CAD build for the part. Positions are in the model's coordinates, mm. Face numbers are marked on the shaded views. Coordinates: 2 decimals unless noted, no trailing zeros. Order: outer loops, then holes, each group sorted by start corner. A loop starts at its lowest first (then second) coordinate and runs counter-clockwise, first axis right, second up. Notation, with made-up numbers: (-15, -2) -> (7, -2) arc R16 cw to (7, 20) -> close; hole circle Ø8 at (0.5, 3). An arc over 180 degrees is marked (long way). Use one line per item in the form item = value. Start each with the question number.
from build123d import *

# Parameters (mm, degrees)
SKETCH_1_W          = 2
SKETCH_1_H          = 2
SKETCH_2_R          = 1
EXTRUDE_1_DEPTH     = 5
CUT_EXTRUDE_1_DEPTH = 1.5
FILLET_1_R          = 0.3


with BuildPart() as part:
    # 草图1 → 旋转1 (revolve)
    with BuildSketch(Plane.XY):
        with Locations((1, -1)):
            Rectangle(SKETCH_1_W, SKETCH_1_H)
    revolve(axis=Axis((0, 0, 0), (0, -1, 0)))

    # 草图2 → 凸台-拉伸1 (add)
    with BuildSketch(Plane.XZ.offset(2)):
        Circle(SKETCH_2_R)
    extrude(amount=EXTRUDE_1_DEPTH)

    # 草图3 → 切除-拉伸1 (cut)
    with BuildSketch(Plane(origin=(0, 0, 0), x_dir=(-1, 0, 0), z_dir=(0, 1, 0))):
        Polygon((0, -0.866025404), (0.75, -0.433012702), (0.75, 0.433012702), (0, 0.866025404), (-0.75, 0.433012702), (-0.75, -0.433012702), align=None)
    extrude(amount=-CUT_EXTRUDE_1_DEPTH, mode=Mode.SUBTRACT)

    # 圆角1
    fillet_1_edges = [part.edges().sort_by_distance(p)[0] for p in [
        (-1, -7, 0),
        (-2, -2, 0),
        (-2, 0, 0),
    ]]
    fillet(fillet_1_edges, radius=FILLET_1_R)


solid = part.part
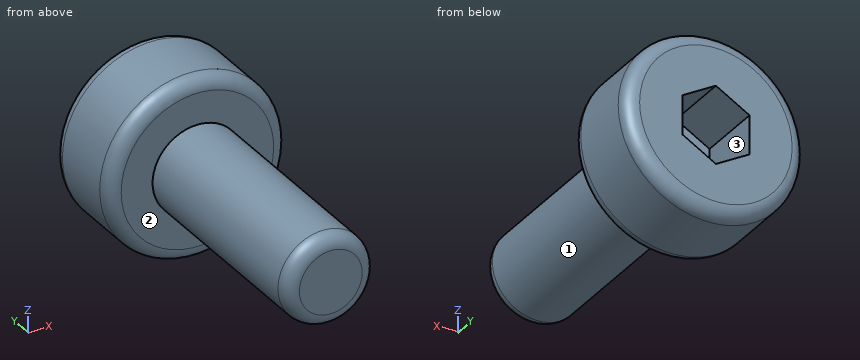
1) Probe L1, parallel to Y at x = -1.45, z = 0.4; L2, parallel to Y at x = -0.45, z = -0.35; L3, parallel to Z at x = -1.05, y = -1. List the from-to ranges inside material, lowest first.
2) Cut at B-B on y = -5. Give the cut face in (x, z).
3) Drop a flat-ended pin along its axis: P1, Ø1, axis at x = 1, y = -6, coming from the +Z side. Give the stop position or say it passes through.
4) Cut at A-A on z = 0. Give the cut face in (x, y).
5) Two-plate mould, pull along X, no slides. Class the marked faces 1, 2 and 3: released by +X, released by -X, zero draft, split by the parting line, or undercut.
Values follow:
q1.L1 = -2 to 0
q1.L2 = -7 to -1.5
q1.L3 = -1.7 to 1.7
q2.outline = circle Ø2 at (0, 0)
q3.P1 = 0.87
q4.outline = (-2, -1.7) arc R0.3 ccw to (-1.7, -2) -> (-1, -2) -> (-1, -6.7) arc R0.3 ccw to (-0.7, -7) -> (0.7, -7) arc R0.3 ccw to (1, -6.7) -> (1, -2) -> (1.7, -2) arc R0.3 ccw to (2, -1.7) -> (2, -0.3) arc R0.3 ccw to (1.7, 0) -> (0.75, 0) -> (0.75, -1.5) -> (-0.75, -1.5) -> (-0.75, 0) -> (-1.7, 0) arc R0.3 ccw to (-2, -0.3) -> close
q5.face_1 = split by the parting line
q5.face_2 = zero draft
q5.face_3 = undercut
